from build123d import *

# Parameters (mm, degrees)
REVOLUTION002_ANGLE  = 180
FILLET006_R          = 0.6
FILLET007_R          = 1
FILLET008_R          = 0.5
SKETCH003_R          = 1
POCKET001_DEPTH      = 0.001
POCKET001_DEPTH_BACK = 5.501


with BuildPart() as part:
    # Sketch004 → Revolution002 (revolve)
    with BuildSketch(Plane.YZ):
        Polygon((-18.5, 2.5), (-13.5, 2.935), (-13.5, 2.5), (-2.5, 2.5), (-2.5, 5.5), (2.5, 5.5), (2.5, 2.5), (13.5, 2.5), (13.5, 2.935), (18.5, 2.5), (18.5, 0), (-18.5, 0), align=None)
    revolve(axis=Axis((0, 0, 0), (0, 1, 0)), revolution_arc=REVOLUTION002_ANGLE)

    # Fillet006
    fillet006_edges = [part.edges().sort_by_distance(p)[0] for p in [
        (2.5, -18.5, 0),
        (2.5, 18.5, 0),
    ]]
    fillet(fillet006_edges, radius=FILLET006_R)

    # Fillet007
    fillet007_edges = [part.edges().sort_by_distance(p)[0] for p in [
        (2.5, -2.5, 0),
        (2.5, 2.5, 0),
    ]]
    fillet(fillet007_edges, radius=FILLET007_R)

    # Fillet008
    fillet008_edges = [part.edges().sort_by_distance(p)[0] for p in [
        (5.5, -2.5, 0),
        (5.5, 2.5, 0),
    ]]
    fillet(fillet008_edges, radius=FILLET008_R)

    # Sketch003 → Pocket001 (cut, two sides)
    with BuildSketch(Plane.YZ) as pocket001_sk:
        Circle(SKETCH003_R)
    extrude(amount=-POCKET001_DEPTH, mode=Mode.SUBTRACT)
    extrude(pocket001_sk.sketch, amount=POCKET001_DEPTH_BACK, mode=Mode.SUBTRACT)


solid = part.part
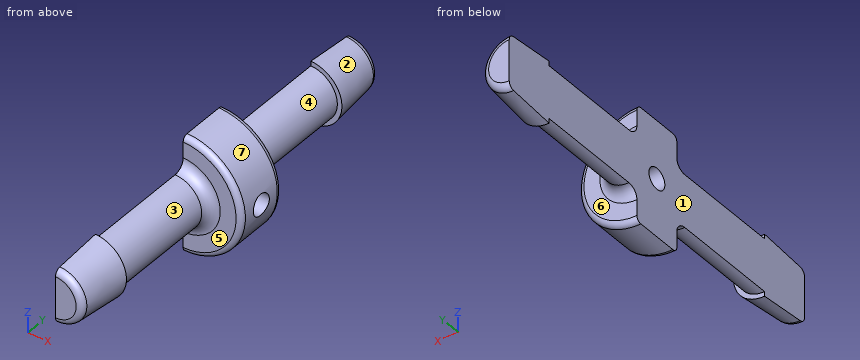
The listing builds one solid part. Answer for the finished solid, in the listing's coordinates (mm). Face numbers are marked on the shaded views. A direction names the side the tool comes from. Round coordinates to 2 decimals unless told otherwise and drop trailing zeros. Order: outer loops, then holes, each group sorted by start corner. A loop starts at its lowest first (then second) coordinate and runs counter-clockwise, first axis right, second up. Notation, with made-up numbers: M -21.75,27.25 L -4.75,27.25 A26 ccw -4.75,44.25 Z; hole C 14.5,74.25 d8. An arc over 180 degrees is marked long. Answer in a Markdown table with one row per item. Add a question column.
1) Flat-ended cylindrical pins translate along their axes: pin 1 Ø6 at (y, z) = (12.5, 1.5) entering from +X (3 decimals); pin 2 Ø1.5 at (x, z) = (4.5, -2) entering from +Y; pin 3 Ø1 at (x, y) = (5, -0.5) entering from +Z. Find the tip coordinate at first contact, or state that the pin passes through.
2) Determine the mould class of the marked faces 1, 2, 3 and 4 for opening direction Y: pulls with the +Y half, pulls with the -Y half, needs draft (parallel to the pull), parting line crosses it, or undercut.
3) The part is cut by section B-B on y = 0. Determine the outline of the cut face in (x, z).
4) The part is cut by section A-A on z = 0. Determine the outline of the cut face in (x, y) (3 decimals), plus the area to 3 significant figures.
5) The part is cut by section C-C on y = -15.5. Determine the outline of the cut face in (x, z), plus the area to 3 significant figures.
6) Which of the six approach directions +Z, -Z, +X, -X, +Y, -Y give full straight-line access (tool end or side, diameter ignored) to the marked faces 5, 6 and 7?
7) Consider line 1 along Y through (x, z) = (1.4, 0); line 2 along Y through (x, z) = (2.1, 4.25); line 3 along Z through (x, y) = (3.45, 0). Determine where each line is inside the solid, lowest interval first. Write a range as from..to.
Findings below:
| question | item | result |
|---|---|---|
| 1 | pin 1 | stops at x = 2.935 |
| 1 | pin 2 | stops at y = 2.5 |
| 1 | pin 3 | stops at z = 3.16 |
| 2 | face 1 | needs draft |
| 2 | face 2 | pulls with the +Y half |
| 2 | face 3 | undercut |
| 2 | face 4 | undercut |
| 3 | outline | M 0,-5.5 A5.5 ccw 5.41,-1 L 0,-1 Z; M 0,1 L 5.41,1 A5.5 ccw 0,5.5 Z |
| 4 | outline | M 0,-18.5 L 1.95,-18.5 A0.6 ccw 2.548,-17.952 L 2.935,-13.5 L 2.5,-13.5 L 2.5,-3.5 A1 cw 3.5,-2.5 L 5,-2.5 A0.5 ccw 5.5,-2 L 5.5,-1 L 0,-1 Z; M 0,1 L 5.5,1 L 5.5,2 A0.5 ccw 5,2.5 L 3.5,2.5 A1 cw 2.5,3.5 L 2.5,13.5 L 2.935,13.5 L 2.548,17.952 A0.6 ccw 1.95,18.5 L 0,18.5 Z |
| 4 | area | 98.9 mm² |
| 5 | outline | M 0,-2.76 A2.76 ccw 0,2.76 Z |
| 5 | area | 12.0 mm² |
| 6 | face 5 | +X, -Y |
| 6 | face 6 | +X, +Y |
| 6 | face 7 | +X, +Y, -Y |
| 7 | line 1 | y = -18.5..-1, 1..18.5 |
| 7 | line 2 | y = -2.5..2.5 |
| 7 | line 3 | z = -4.28..-1, 1..4.28 |
